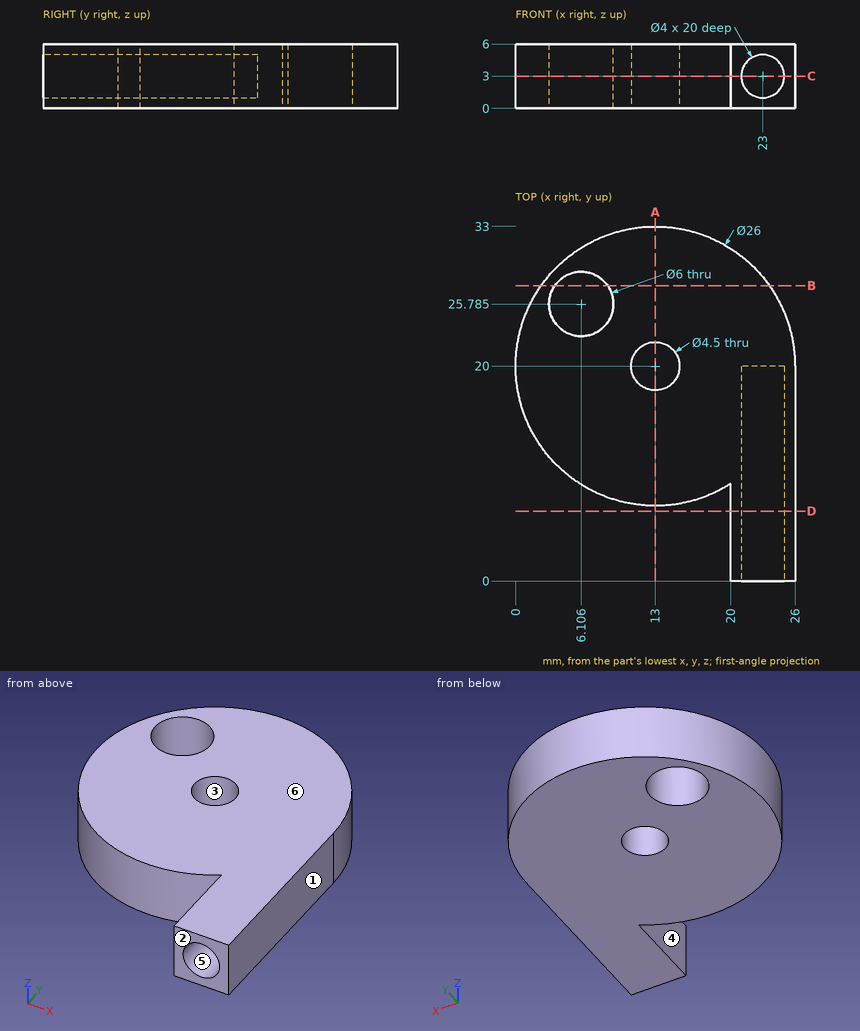
Check sheet for the drawn part. Datum: minimum x, y, z corner. Units: mm. A direction names the side the tool comes from. Coordinates: 2 decimals unless noted, no trailing zeros. Loops run counter-clockwise (first coordinate to the right, second up) from the corner with the lowest first, then second, coordinate; pieces in that order, holes last. Notation, with made-up numbers: M -3.75,50.25 L 19.25,50.25 A32 cw 19.25,85.25 Z; hole C 52,-21 d4. An arc over 180 degrees is marked long. Answer as a JSON object with one key per item and string values.
1. Access from +Z, -Z, +X, -X, +Y, -Y to the whole of each face (thin tool, end or side, straight path). Record for the marked faces 4, 5 and 6.
Outcome:
{"face 4": "+Z, -Z, -Y", "face 5": "-Y", "face 6": "+Z, +X, -X, +Y, -Y"}
2. Sectioned sample at D-D on y = 6.5. Record the cut outline in (x, z).
Outcome:
{"outline": "M 20,0 L 26,0 L 26,6 L 20,6 Z; hole C 23,3 d4"}
3. Scan lines: L1, parallel to X at y = 6.75, z = 3; L2, parallel to Y at x = 25, z = 1.35; L3, parallel to X at y = 12, z = 4.05 (1 decimal). Record each from-to range of solid material in increasing order. Write a range as from..to.
Outcome:
{"L1": "20..21, 25..26", "L2": "0..25", "L3": "2.8..21.3, 24.7..26"}
4. Sectioned sample at C-C on z = 3. Count the separate pieces of the cut face and the enclosed holes in it.
Outcome:
{"separate pieces": "1", "enclosed holes": "2"}
5. Depth check by flat-ended pin: P1, Ø3, axis at x = 23, z = 3, coming from the -Y side; P2, Ø4, axis at x = 13, y = 20, coming from the -Z side; P3, Ø3, axis at x = 4, z = 3.5, coming from the +Y side; P4, Ø1, axis at x = 14.5, z = 3, coming from the -Y side. Enter the tip coordinate at first touch or a pass-through.
Outcome:
{"P1": "y = 20", "P2": "through", "P3": "y = 30.62", "P4": "y = 7.04"}
6. Release check for a two-part mould opening along X. For the marked faces 1, 2 and 3 record: pulls with the +X half, pulls with the -X half, needs draft (parallel to the pull), parting line crosses it, or undercut.
Outcome:
{"face 1": "pulls with the +X half", "face 2": "needs draft", "face 3": "undercut"}
7. Sectioned sample at A-A on x = 13. Record the cut outline in (y, z), and give its area (3 significant figures).
Outcome:
{"outline": "M 7,0 L 17.75,0 L 17.75,6 L 7,6 Z; M 22.25,0 L 33,0 L 33,6 L 22.25,6 Z", "area": "129 mm²"}
8. Sectioned sample at B-B on y = 27.5. Record the cut outline in (x, z).
Outcome:
{"outline": "M 2.38,0 L 3.64,0 L 3.64,6 L 2.38,6 Z; M 8.57,0 L 23.62,0 L 23.62,6 L 8.57,6 Z"}
